Verification items for the finished model (mm, model axes). Face numbers are marked on the shaded views. A direction names the side the tool comes from. Give positions to 0.01 mm unless a question says otherwise; leave off trailing zeros. Answer as CSV lines item,"result".
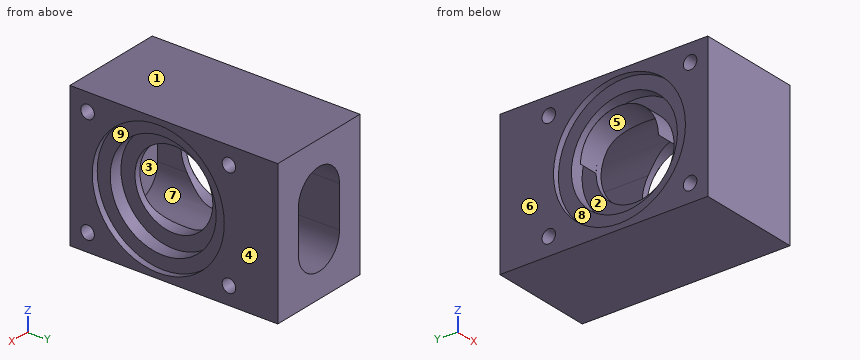
Autodesk Inventor part; units mm, degrees
ref_plane "YZ Plane" through (0, 0, 0) normal (1, 0, 0) x (0, 1, 0)
ref_plane "XZ Plane" through (0, 0, 0) normal (0, 1, 0) x (-1, 0, 0)
ref_plane "XY Plane" through (0, 0, 0) normal (0, 0, 1) x (1, 0, 0)
sketch "Sketch1" plane through (0, 0, 0) normal (0, 1, 0) x (-1, 0, 0)
  line L0 (0, 0) -> (25.4, 0)
  line L1 (25.4, 0) -> (25.4, -34.925)
  line L2 (25.4, -34.925) -> (0, -34.925)
  line L3 (0, -34.925) -> (0, 0)
  dimension "BlockW" = 25.4
  dimension "BlockL" = 34.925
extrude "Extrusion1" add sketch "Sketch1" along normal blind 50.8
sketch "Sketch2" plane through (0, 50.8, 0) normal (0, 1, 0) x (1, 0, 0)
  line L0 (0, 0) -> (-12.7, 0)
  line L1 (0, 17.4625) -> (0, 0)
  line L2 (-12.7, 22.5425) -> (-12.7, 12.3825) construction
  line L3 (-19.05, 22.5425) -> (-19.05, 12.3825)
  line L4 (-6.35, 12.3825) -> (-6.35, 22.5425)
  arc A0 (-6.35, 22.5425) -> (-19.05, 22.5425) centre (-12.7, 22.5425) ccw
  arc A1 (-19.05, 12.3825) -> (-6.35, 12.3825) centre (-12.7, 12.3825) ccw
  line L5 (-12.7, 17.4625) -> (-2.54, 17.4625) construction
  dimension "d4" = 12.7
  dimension "d5" = 17.4625
  dimension "d33" = 5.08
  dimension "d35" = 12.7
extrude "Extrusion7" cut sketch "Sketch2" against normal blind 44.45
sketch "Sketch3" plane through (0, 0, 0) normal (1, 0, 0) x (0, 0, -1)
  line L0 (0, 0) -> (17.4752, 0)
  line L1 (0, 21.59) -> (0, 0)
  circle A0 centre (17.4752, 21.59) radius 9.525
  circle A1 centre (17.4752, 21.59) radius 12.954
  circle A2 centre (17.4752, 21.59) radius 16.129
  line L2 (4.318, 21.59) -> (21.59, 21.59) construction
  point P0 (4.318, 38.862)
  dimension "d15" = 19.05
  dimension "d16" = 25.908
  dimension "d17" = 32.258
hole "Hole2" at (0, 38.862, -4.318) direction (-1, 0, 0) diameter 3.302 depth 10.16
pattern_linear "Rectangular Pattern1" count 2 spacing 26.289 along (0, 0, -1) count 2 spacing 34.544 along (0, -1, 0) of "Hole2"
extrude "Extrusion2" cut sketch "Sketch3" against normal through all contours A0
extrude "Extrusion3" cut sketch "Sketch3" against normal blind 4.826 contours A1
extrude "Extrusion4" cut sketch "Sketch3" against normal blind 1.524 contours A2
sketch "Sketch4" plane through (-25.4, 0, -34.925) normal (-1, 0, 0) x (0, 0, 1)
  line L0 (0, 0) -> (17.4752, 0)
  line L1 (17.4752, 21.59) -> (0, 21.59)
  line L2 (0, 21.59) -> (0, 0)
  circle A0 centre (17.4752, 21.59) radius 9.525
  circle A1 centre (17.4752, 21.59) radius 12.954
  circle A2 centre (17.4752, 21.59) radius 16.129
  line L3 (17.4752, 21.59) -> (30.6197, 21.59)
  line L4 (30.6197, 21.59) -> (30.6197, 38.862)
  line L5 (30.6197, 38.862) -> (17.4752, 38.862)
  line L6 (17.4752, 38.862) -> (17.4752, 21.59)
  point P0 (34.925, 0)
  dimension "d24" = 17.4752
  dimension "d25" = 21.59
  dimension "d26" = 19.05
  dimension "d28" = 32.258
  dimension "d57" = 13.1445
  dimension "d58" = 17.272
extrude "Extrusion5" cut sketch "Sketch4" against normal blind 4.826 contours A0 L3 A1 L1 | L1 A1 L6 A0 | A0 L6 A1 L3
extrude "Extrusion6" cut sketch "Sketch4" against normal blind 1.524 contours A1 L3 L4 A2 L1 | L1 A2 L6 A1 | A1 L6 A2 L4 L3
hole "Hole3" at (-25.4, 38.862, -4.3053) direction (1, 0, 0) diameter 3.302 depth 10.16
pattern_linear "Rectangular Pattern2" count 2 spacing 26.289 along (0, 0, -1) count 2 spacing 34.544 along (0, -1, 0) of "Hole3"
equation "\"d4\" = 0.5 * BlockW"
equation "\"d5\" = 0.5 * BlockL"
equation "\"d36\" = WellDepth"
properties part number "VaporFlowBlock"
1) Depth check by flat-ended pin: pin 1 (2.5 mm diameter, centred on y = 4.318, z = -4.318, fed in from +X); pin 2 (10 mm diameter, centred on x = -13, z = -16.5, fed in from +Y); pin 3 (1.7 mm diameter, centred on y = 39, z = -30.5, fed in from -X). Enter the tip coordinate at first touch or a pass-through.
Reported:
pin 1,"x = -10.16"
pin 2,"y = 6.35"
pin 3,"x = -15.24"
2) Tool access check on the marked faces 5, 6, 7, 8 and 9. Record the directions out of +Z, -Z, +X, -X, +Y, -Y that give a thin tool (end or side, any length) a straight path to the whole face; none if there is none.
Reported:
face 5,"+X, -X"
face 6,"+Z, -Z, -X, +Y, -Y"
face 7,"+Y"
face 8,"-X"
face 9,"+X"
3) Scan lines: line 1 along X through (y, z) = (41, -27); line 2 along Y through (x, z) = (-5.25, -3); line 3 along Y through (x, z) = (-3.5, -31.5). Record each from-to range of solid material in increasing order.
Reported:
line 1,"-25.4 to -17.22, -8.18 to 0"
line 2,"0 to 3.32, 5.31 to 37.87, 39.86 to 50.8"
line 3,"0 to 2.93, 5.71 to 37.47, 40.25 to 50.8"
4) Section check A-A (z = -18). State how many separate pieces and enclosed holes the cut face has, and give its area (3 significant figures).
Reported:
separate pieces,"3"
enclosed holes,"0"
area,"399 mm²"
5) Draft check along X on the marked faces 1, 2, 3 and 4. Enter one of: +X half, -X half, draft (parallel to the pull), parting line (faces both ways), or undercut.
Reported:
face 1,"draft"
face 2,"-X half"
face 3,"undercut"
face 4,"+X half"
